Part model, mm, in its own coordinate system. A direction names the side the tool comes from. Coordinates: 2 decimals unless noted, no trailing zeros. Loops run counter-clockwise (first coordinate to the right, second up) from the corner with the lowest first, then second, coordinate; pieces in that order, holes last. Notation, with made-up numbers: (55, 36) - (104, 36) arc R12 cw to (104, 47) - close; hole circle Ø2 at (75.5, 33). An arc over 180 degrees is marked (long way). Use a Markdown table: item, result. Add a question column.
1. Wall check: probe 1 along X at (y, z) = (1.65, -51.5); probe 2 along Z at (x, y) = (20.5, 2.65); probe 3 along Z at (x, y) = (6.5, 2). Give the ranges that are in metal, low to high. Write a range as [from, to].
2. Band-saw the part on D-D, the plane x = 15. Give the cut face in (y, z), plus the area to 3 significant figures.
3. Band-saw the part on A-A, the plane x = 6. Give the cut face in (y, z).
4. 3-axis set-ups, long thin cutter, end or side, ignore diameter. For faces 4 (the flat face through (12, 1, -63)), 5 (the flat face through (6, 1, -64.5)), 6 (the flat face through (32, 1, -29)): which of +Z, -Z, +X, -X, +Y, -Y reach the whole face in a straight line?
5. Band-saw the part on C-C, the plane z = -51.5. Give the cut face in (x, y).
6. Pull direction X, two halves, no side cores. Call faces 1 (the flat face through (4, 1, -64)), 2 (the flat face through (22, 1, -58)), 3 (the flat face through (0, 1, -34)): pulls with the +X half, pulls with the -X half, needs draft (parallel to the pull), parting line crosses it, or undercut.
7. Band-saw the part on B-B, the plane y = 2.25. Give the cut face in (x, z).
8. Drop flat-ended pins along their axis: pin 1 (1.5 mm diameter, centred on x = 22, y = 1, fed in from -Z); pin 2 (1.6 mm diameter, centred on y = 1, z = -64, fed in from +X); pin 3 (2 mm diameter, centred on x = 26.5, z = -16, fed in from -Y). Give the stop position or say it passes through.
from build123d import *

# Parameters (mm, degrees)
SKETCH1_R           = 1.5
SKETCH1_W           = 4
SKETCH1_H           = 1.5
BOSS_EXTRUDE1_DEPTH = 3
SKETCH3_W           = 12
SKETCH3_H           = 3
CUT_EXTRUDE2_DEPTH  = 82.049367672


with BuildPart() as part:
    # Sketch1 → Boss-Extrude1 (new body)
    with BuildSketch(Plane(origin=(0, 0, 0), x_dir=(1, 0, 0), z_dir=(0, 1, 0))):
        Polygon((0, 58), (0, 68), (12, 68), (12, 58), (44, 58), (44, 0), (0, 0), align=None)
        with Locations(Location((20, 51.5, 0), (0, 0, 270))):
            Circle(SKETCH1_R, mode=Mode.SUBTRACT)
        with Locations(Location((36, 51.5, 0), (0, 0, 270))):
            Circle(SKETCH1_R, mode=Mode.SUBTRACT)
        with Locations((6, 63.75)):
            Rectangle(SKETCH1_W, SKETCH1_H, mode=Mode.SUBTRACT)
    extrude(amount=BOSS_EXTRUDE1_DEPTH)

    # Sketch3 → Cut-Extrude2 (cut, through all)
    with BuildSketch(Plane.XY):
        with Locations((38, 1.5)):
            Rectangle(SKETCH3_W, SKETCH3_H)
    extrude(amount=-CUT_EXTRUDE2_DEPTH, mode=Mode.SUBTRACT)


solid = part.part
Geometry check:
| question | item | result |
|---|---|---|
| 1 | probe 1 | x = [0, 18.5], [21.5, 32] |
| 1 | probe 2 | z = [-58, -52.91], [-50.09, 0] |
| 1 | probe 3 | z = [-68, -64.5], [-63, 0] |
| 2 | outline | (0, -58) - (3, -58) - (3, 0) - (0, 0) - close |
| 2 | area | 174 mm^2 |
| 3 | outline | (0, -68) - (3, -68) - (3, -64.5) - (0, -64.5) - close; (0, -63) - (3, -63) - (3, 0) - (0, 0) - close |
| 4 | face 4 | -Z, +X, +Y, -Y |
| 4 | face 5 | +Y, -Y |
| 4 | face 6 | +Z, -Z, +X, +Y, -Y |
| 5 | outline | (0, 0) - (18.5, 0) - (18.5, 3) - (0, 3) - close; (21.5, 0) - (32, 0) - (32, 3) - (21.5, 3) - close |
| 6 | face 1 | undercut |
| 6 | face 2 | needs draft |
| 6 | face 3 | pulls with the -X half |
| 7 | outline | (0, -68) - (12, -68) - (12, -58) - (32, -58) - (32, 0) - (0, 0) - close; hole (4, -64.5) - (8, -64.5) - (8, -63) - (4, -63) - close; hole circle Ø3 at (20, -51.5) |
| 8 | pin 1 | stops at z = -58 |
| 8 | pin 2 | stops at x = 12 |
| 8 | pin 3 | stops at y = 0 |
